Part model, mm, in its own coordinate system. A direction names the side the tool comes from. Give positions to 0.01 mm unless a question says otherwise; leave off trailing zeros. Loops run counter-clockwise (first coordinate to the right, second up) from the corner with the lowest first, then second, coordinate; pieces in that order, holes last. Notation, with made-up numbers: M 71.25,-23.5 L 87.25,-23.5 A13 cw 87.25,-7.5 Z; hole C -27,80 d11. An arc over 180 degrees is marked long. Answer in a Markdown table with one row per item.
Autodesk Inventor part; units mm, degrees
ref_plane "YZ Plane" through (0, 0, 0) normal (1, 0, 0) x (0, 1, 0)
ref_plane "XZ Plane" through (0, 0, 0) normal (0, 1, 0) x (-1, 0, 0)
ref_plane "XY Plane" through (0, 0, 0) normal (0, 0, 1) x (1, 0, 0)
sketch "Sketch1" plane through (0, 0, 0) normal (0, 1, 0) x (-1, 0, 0)
  circle A0 centre (0, 0) radius 3.175
  circle A1 centre (0, 0) radius 4.9147
  dimension "BoreD" = 6.35
  dimension "OuterD" = 9.8294
extrude "Extrusion1" add sketch "Sketch1" along normal blind 9
sketch "Sketch2" plane through (0, 0, 0) normal (0, -1, 0) x (1, 0, 0)
  circle A0 centre (0, 0) radius 4.9147
  arc A1 (0.4982, -4.7076) -> (0.668, -4.8691) centre (0.6476, -4.7205) ccw
  arc A2 (0.4982, -4.7076) -> (-0.4982, -4.7076) centre (0, -4.6647) ccw
  arc A3 (-0.668, -4.8691) -> (-0.4982, -4.7076) centre (-0.6476, -4.7205) ccw
  point P0 (0, -4.9147)
  dimension "d9" = 0.5
  dimension "d10" = 0.15
  dimension "Depth" = 0.25
extrude "Extrusion2" cut sketch "Sketch2" against normal up to next contours A3 A2 A1 A0 picked at (0, -4.6613)
pattern_circular "Circular Pattern1" count 16 over 360 about axis through (0, -10, 0) along (0, 1, 0) of "Extrusion2"
sketch "Sketch3" plane through (0, 0, 0) normal (0, -1, 0) x (1, 0, 0)
  circle A0 centre (0, 0) radius 5.7897
  circle A1 centre (0, 0) radius 3.175
  dimension "FaceD" = 11.5794
  dimension "d18" = 6.35
extrude "Extrusion3" add sketch "Sketch3" along normal blind 1.5
sketch "Sketch4" plane through (0, 9, 0) normal (0, 1, 0) x (1, 0, 0)
  circle A0 centre (0, 0) radius 3.175
  circle A1 centre (0, 0) radius 5.175
  circle A2 centre (0, 0) radius 5.7897
  dimension "d21" = 2
extrude "Extrusion4" [suppressed]
extrude "Extrusion5" add sketch "Sketch4" along normal blind 6 contours A1
sketch "Sketch5" plane through (0, 0, 0) normal (1, 0, 0) x (0, 1, 0)
  circle A0 centre (12, 0) radius 1.5
  line L0 (9, -5.175) -> (15, -5.175)
  point P0 (0, 0)
  point P1 (12, -5.175)
  dimension "d26" = 3
extrude "Extrusion6" cut sketch "Sketch5" along normal through all both and the other way through all
equation "\"OuterD\" = 0.0614338 * Teeth"
equation "\"d18\" = BoreD"
equation "\"BeltWidth\" = 8"
equation "\"Pitch\" = 0.25"
properties part number "GT2Shaft16T" material "ABS Plastic"
(1) Saw through at D-D (z = -1.75). Write the cut outline in (x, y), plus the area to 3 significant figures.
Recorded:
| item | result |
|---|---|
| outline | M -5.52,-1.5 L -2.65,-1.5 L -2.65,15 L -4.87,15 L -4.87,9 L -3.81,9 L -3.81,0 L -5.52,0 Z; M 2.65,-1.5 L 5.52,-1.5 L 5.52,0 L 3.81,0 L 3.81,9 L 4.87,9 L 4.87,15 L 2.65,15 Z |
| area | 56.2 mm^2 |
(2) Which spindle directions (+Z, -Z, +X, -X, +Y, -Y) get a long thin tool onto all of the face, cutting with end or side? Do faces 4 (the face through (4.78, 11.96, -1.98)), 5 (the face through (3.97, 10.5, -0.07)), 6 (the face through (-3.852, 4.437, 1.583)). Say none if no direction does.
Recorded:
| item | result |
|---|---|
| face 4 | +Y |
| face 5 | +X, -X |
| face 6 | none |
(3) Pin check, flat tip, straight feed: pin 1 Ø4 at (x, y) = (1.5, 3.5) entering from -Z. Stop position of the tip, or through.
Recorded:
| item | result |
|---|---|
| pin 1 | stops at z = -4.87 |
(4) Saw through at C-C (y = 12). Write the cut outline in (x, z) (3 decimals).
Recorded:
| item | result |
|---|---|
| outline | M -4.953,-1.5 A5.175 ccw 4.953,-1.5 L 2.798,-1.5 A3.175 cw -2.798,-1.5 Z; M -4.953,1.5 L -2.798,1.5 A3.175 cw 2.798,1.5 L 4.953,1.5 A5.175 ccw Z |
(5) Drill centre lines: line 1 along Y through (x, z) = (0, -4.25); line 2 along X through (y, z) = (1.5, 4); line 3 along Z through (x, y) = (0.5, 13.25). Where is each one in solid material? Low to high.
Recorded:
| item | result |
|---|---|
| line 1 | y = -1.5 to 0, 9 to 15 |
| line 2 | x = -2.86 to -2.18, -1.39 to 1.39, 2.18 to 2.86 |
| line 3 | z = -5.15 to -3.14, 3.14 to 5.15 |
(6) Saw through at B-B (z = 0). Write the cut outline in (x, y) (3 decimals), plus the area to 3 significant figures.
Recorded:
| item | result |
|---|---|
| outline | M -5.79,-1.5 L -3.175,-1.5 L -3.175,10.5 L -5.175,10.5 L -5.175,9 L -4.165,9 L -4.165,0 L -5.79,0 Z; M -5.175,13.5 L -3.175,13.5 L -3.175,15 L -5.175,15 Z; M 3.175,-1.5 L 5.79,-1.5 L 5.79,0 L 4.165,0 L 4.165,9 L 5.175,9 L 5.175,10.5 L 3.175,10.5 Z; M 3.175,13.5 L 5.175,13.5 L 5.175,15 L 3.175,15 Z |
| area | 37.7 mm^2 |
(7) Pull direction X, two halves, no side cores. Call faces 1 (the face through (-0.1, 15, 3.4)), 2 (the face through (1.583, 4.437, 3.852)), 3 (the face through (3.113, -0.74, -4.882)): +X half, -X half, draft (parallel to the pull), parting line (faces both ways), or undercut.
Recorded:
| item | result |
|---|---|
| face 1 | draft |
| face 2 | undercut |
| face 3 | parting line |
(8) Saw through at A-A (x = 0). Write the cut outline in (y, z) (3 decimals).
Recorded:
| item | result |
|---|---|
| outline | M -1.5,-5.79 L 0,-5.79 L 0,-4.165 L 9,-4.165 L 9,-5.175 L 15,-5.175 L 15,-3.175 L -1.5,-3.175 Z; M -1.5,3.175 L 15,3.175 L 15,5.175 L 9,5.175 L 9,4.165 L 0,4.165 L 0,5.79 L -1.5,5.79 Z |
